```python
from build123d import *

# Parameters (mm, degrees)
SKETCH052_W       = 10.2
SKETCH052_H       = 10.2
PAD044_DEPTH      = 4
PAD044_DEPTH_BACK = 2
SKETCH053_R       = 2
POCKET004_DEPTH   = 1
CHAMFER006_SIZE2  = 2
CHAMFER006_SIZE   = 0.5
SKETCH049_W       = 4.3
SKETCH049_H       = 5
POCKET006_DEPTH   = 5


with BuildPart() as part:
    # Sketch052 (on Face1 of CopyFillet001) → Pad044 (new body, two sides)
    with BuildSketch(Plane(origin=(0, 9, 0), x_dir=(-1, 0, 0), z_dir=(0, 1, 0))) as pad044_sk:
        with Locations((0, 2)):
            Rectangle(SKETCH052_W, SKETCH052_H)
    extrude(amount=PAD044_DEPTH)
    extrude(pad044_sk.sketch, amount=-PAD044_DEPTH_BACK)

    # Sketch053 (on Face1 of Pad044) → Pocket004 (cut)
    with BuildSketch(Plane(origin=(0, 9, 7.1), x_dir=(1, 0, 0), z_dir=(0, 0, 1))):
        with Locations((-2.5, 1)):
            Circle(SKETCH053_R)
        with Locations((2.5, 1)):
            Circle(SKETCH053_R)
    extrude(amount=-POCKET004_DEPTH, mode=Mode.SUBTRACT)

    # Chamfer006
    chamfer006_edges = [part.edges().sort_by_distance(p)[0] for p in [
        (0, 13, 7.1),
    ]]
    chamfer006_side = part.faces().sort_by_distance((0, 10, 7.1))[0]
    chamfer(chamfer006_edges, length=CHAMFER006_SIZE, length2=CHAMFER006_SIZE2, reference=chamfer006_side)

    # Sketch049 (on Face8 of Chamfer006) → Pocket006 (cut)
    with BuildSketch(Plane(origin=(0, 13, 0), x_dir=(-1, 0, 0), z_dir=(0, 1, 0))):
        with Locations((-2.65, 0)):
            Rectangle(SKETCH049_W, SKETCH049_H)
        with Locations((2.65, 0)):
            Rectangle(SKETCH049_W, SKETCH049_H)
    extrude(amount=-POCKET006_DEPTH, mode=Mode.SUBTRACT)


solid = part.part
```
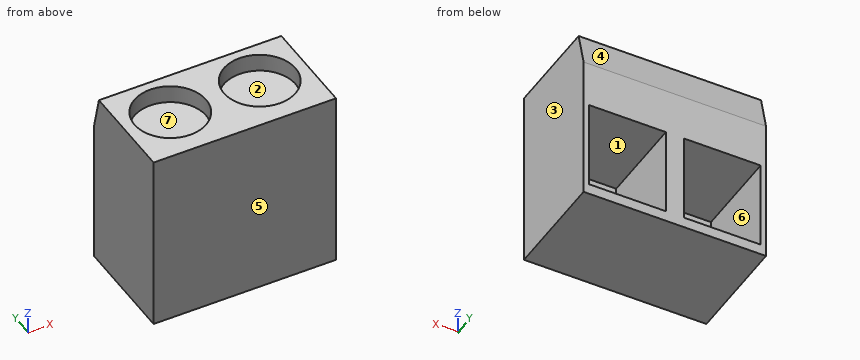
Design review of the part built by this model. Coordinates are the model's own, in mm. Face numbers are marked on the shaded views. A direction names the side the tool comes from. Give positions to 0.01 mm unless a question says otherwise; leave off trailing zeros. Loops run counter-clockwise (first coordinate to the right, second up) from the corner with the lowest first, then second, coordinate; pieces in that order, holes last. Notation, with made-up numbers: M 25.25,78.5 L 56.25,78.5 A24 ccw 56.25,104.5 Z; hole C -31.75,31.5 d10. An arc over 180 degrees is marked long. Return JSON: item names as keys, results as strings. Group by question number.
Item 1: We need section B-B (z = 0). Give the boundary of the cut face in (x, y), and give its area (3 significant figures).
Item 2: For probe 1 along X at (y, z) = (10.4, 1); probe 2 along Z at (x, y) = (4, 8.5); probe 3 along Z at (x, y) = (-1, 9.85), list the stretches that pass through material, from the lowest coordinate up.
Item 3: Tool access review of the marked faces 1, 2 and 3: name each direction out of +Z, -Z, +X, -X, +Y, -Y from which nothing blocks a thin tool from reaching the whole face with its end or side.
Item 4: We need section A-A (y = 10). Give the boundary of the cut face in (x, z), and give its area (3 significant figures).
Item 5: We need section D-D (x = 3.75). Give the boundary of the cut face in (y, z).
Item 6: We need section C-C (x = 2.5). Give the boundary of the cut face in (y, z), and give its area (3 significant figures).
Item 7: Mouldability with a two-part tool opening along Y and no side actions: class the marked faces 4, 5, 6 and 7 as released by +Y, released by -Y, zero draft, split by the parting line, or undercut.
Item 8: Insertion check: pin 1 Ø2.5 at (x, y) = (-2.5, 10) entering from +Z; pin 2 Ø2 at (x, z) = (2.5, 0.5) entering from +Y. Each pin has a flat end and moves straight along its axis. Give the tip position at first contact, or say it passes through.
Output:
{
 "1": {"outline": "M -5.1,7 L 5.1,7 L 5.1,13 L 4.8,13 L 4.8,8 L 0.5,8 L 0.5,13 L -0.5,13 L -0.5,8 L -4.8,8 L -4.8,13 L -5.1,13 Z", "area": "18.2 mm^2"},
 "2": {"probe 1": "x = -5.1 to -4.8, -0.5 to 0.5, 4.8 to 5.1", "probe 2": "z = -3.1 to -2.5, 2.5 to 7.1", "probe 3": "z = -3.1 to -2.5, 2.5 to 6.1"},
 "3": {"face 1": "+Y", "face 2": "+Z", "face 3": "+Z, -Z, +X, +Y, -Y"},
 "4": {"outline": "M -5.1,-3.1 L 5.1,-3.1 L 5.1,7.1 L 4.5,7.1 L 4.5,6.1 L 0.5,6.1 L 0.5,7.1 L -0.5,7.1 L -0.5,6.1 L -4.5,6.1 L -4.5,7.1 L -5.1,7.1 Z; hole M -4.8,-2.5 L -0.5,-2.5 L -0.5,2.5 L -4.8,2.5 Z; hole M 0.5,-2.5 L 4.8,-2.5 L 4.8,2.5 L 0.5,2.5 Z", "area": "53.0 mm^2"},
 "5": {"outline": "M 7,-3.1 L 13,-3.1 L 13,-2.5 L 8,-2.5 L 8,2.5 L 13,2.5 L 13,5.1 L 12.5,7.1 L 11.56,7.1 L 11.56,6.1 L 8.44,6.1 L 8.44,7.1 L 7,7.1 Z"},
 "6": {"outline": "M 7,-3.1 L 13,-3.1 L 13,-2.5 L 8,-2.5 L 8,2.5 L 13,2.5 L 13,5.1 L 12.5,7.1 L 12,7.1 L 12,6.1 L 8,6.1 L 8,7.1 L 7,7.1 Z", "area": "31.7 mm^2"},
 "7": {"face 4": "released by +Y", "face 5": "released by -Y", "face 6": "zero draft", "face 7": "undercut"},
 "8": {"pin 1": "stops at z = 6.1", "pin 2": "stops at y = 8"}
}
